Check sheet for the modelled part. Datum: model origin and axes. Units: mm. A direction names the side the tool comes from. Round coordinates to 2 decimals unless told otherwise and drop trailing zeros. Write each loop counter-clockwise with the first axis right and the second up, starting at its lowest first coordinate (ties: lowest second). Pieces come first, ordered by that corner, then holes.
from build123d import *

# Parameters (mm, degrees)
BOSS_EXTRUDE1_DEPTH = 3
CUT_EXTRUDE1_DEPTH  = 18


with BuildPart() as part:
    # Sketch1 → Revolve1 (revolve)
    with BuildSketch(Plane(origin=(0, 0, 0), x_dir=(1, 0, 0), z_dir=(0, 1, 0))):
        with BuildLine():
            Line((7.15, 0), (6.125, 0))
            Line((6.125, 0), (6.125, -10))
            Line((6.125, -10), (5.77, -10.204959346))
            Line((5.77, -10.204959346), (5.77, -18))
            Line((5.77, -18), (0, -18))
            Line((0, -18), (0, 6.1))
            ThreePointArc((0, 6.1), (2.269911893, 5.949339194), (4.5, 5.5))
            Line((4.5, 5.5), (4.5, 2.5))
            Line((4.5, 2.5), (6.15, 2.5))
            Line((6.15, 2.5), (7.15, 1.5))
            Line((7.15, 1.5), (7.15, 0))
        make_face()
    revolve(axis=Axis((0, 0, -49.656832942), (0, 0, 1)))

    # Sketch2 → Boss-Extrude1 (add)
    with BuildSketch(Plane.XY.offset(18)):
        with BuildLine():
            Line((2.6, -0.45), (2.6, 0.45))
            ThreePointArc((2.6, 0.45), (3.5, 1.35), (4.4, 0.45))
            Line((4.4, 0.45), (4.4, -0.45))
            ThreePointArc((4.4, -0.45), (3.5, -1.35), (2.6, -0.45))
        make_face()
    boss_extrude1 = extrude(amount=BOSS_EXTRUDE1_DEPTH)

    # Mirror1: Boss-Extrude1 across plane
    add(boss_extrude1.mirror(Plane(origin=(0, 0, 0), x_dir=(0, 0, 1), z_dir=(1, 0, 0))))

    # Sketch3 → Cut-Extrude1 (cut)
    with BuildSketch(Plane.XY.offset(18)):
        with BuildLine():
            Line((5.75, 2.110242877), (5.75, -2.110242877))
            ThreePointArc((5.75, -2.110242877), (6.125, 0), (5.75, 2.110242877))
        make_face()
        with BuildLine():
            Line((-5.75, 2.110242877), (-5.75, -2.110242877))
            ThreePointArc((-5.75, -2.110242877), (-6.125, 0), (-5.75, 2.110242877))
        make_face()
    extrude(amount=-CUT_EXTRUDE1_DEPTH, mode=Mode.SUBTRACT)


solid = part.part
1. Go/stop test with flat-tipped pins: pin 1 (3.5 mm diameter, centred on x = -2, y = 1.5, fed in from -Z); pin 2 (1.5 mm diameter, centred on x = 5, y = -4, fed in from -Z); pin 3 (0.5 mm diameter, centred on y = 0, z = 19.5, fed in from +X). Record where each tip stops, or that it passes through.
2. Sectioned sample at A-A, the plane x = 0. Enter the section's corners in (y, z) (3 decimals).
3. Set-up check for faces 1 (the flat face through (5.75, 0, 7)), 2 (the flat face through (0, -5, -2.5)), 3 (the cylindrical face through (0.105, 6.124, 5.07)), 4 (the flat face through (2.6, 0, 19)): record each of +Z, -Z, +X, -X, +Y, -Y from which the full face is reachable in a straight line by a thin tool's end or side.
4. Scan lines: line 1 along Z through (x, y) = (-1, 5.25); line 2 along X through (y, z) = (2, 10); line 3 along Z through (x, y) = (5.5, 3.5). Record each from-to range of solid material in increasing order.
5. Sectioned sample at D-D, the plane z = 17.25. Enter the section's corners in (x, y).
6. Sectioned sample at C-C, the plane z = 7.75. Enter the section's corners in (x, y) (3 decimals).
7. Sectioned sample at B-B, the plane y = 0. Enter the section's corners in (x, z) (3 decimals).
Computed values:
1. pin 1: stops at z = -6.08
1. pin 2: stops at z = -2.5
1. pin 3: stops at x = 4.4
2. outline: (-7.15, -1.5) - (-6.15, -2.5) - (-4.5, -2.5) - (-4.5, -5.5) arc R17.175 ccw to (4.5, -5.5) - (4.5, -2.5) - (6.15, -2.5) - (7.15, -1.5) - (7.15, 0) - (6.125, 0) - (6.125, 10) - (5.77, 10.205) - (5.77, 18) - (-5.77, 18) - (-5.77, 10.205) - (-6.125, 10) - (-6.125, 0) - (-7.15, 0) - close
3. face 1: +Z, +X, +Y, -Y
3. face 2: -Z
3. face 3: +Z, +Y
3. face 4: +Z, +Y, -Y
4. line 1: z = -2.5 to 18
4. line 2: x = -5.75 to 5.75
4. line 3: z = -2.13 to 0
5. outline: (-5.75, -0.48) arc R5.77 ccw to (5.75, -0.48) - (5.75, 0.48) arc R5.77 ccw to (-5.75, 0.48) - close
6. outline: (-5.75, -2.11) arc R6.125 ccw to (5.75, -2.11) - (5.75, 2.11) arc R6.125 ccw to (-5.75, 2.11) - close
7. outline: (-7.15, -1.5) - (-6.15, -2.5) - (-4.5, -2.5) - (-4.5, -5.5) arc R17.175 ccw to (4.5, -5.5) - (4.5, -2.5) - (6.15, -2.5) - (7.15, -1.5) - (7.15, 0) - (5.75, 0) - (5.75, 18) - (4.4, 18) - (4.4, 21) - (2.6, 21) - (2.6, 18) - (-2.6, 18) - (-2.6, 21) - (-4.4, 21) - (-4.4, 18) - (-5.75, 18) - (-5.75, 0) - (-7.15, 0) - close
